from build123d import *

# Parameters (mm, degrees)
SKETCH2_R                        = 9.525
SKETCH2_R_2                      = 4.7625
BOSS_EXTRUDE1_DEPTH              = 19.05
SKETCH2_3_R                      = 4.7625
BOSS_EXTRUDE2_DEPTH              = 19.05
F_5_8_0_625_DIAMETER_HOLE1_D     = 15.875
F_5_8_0_625_DIAMETER_HOLE1_DEPTH = 14.280668836
F_5_8_0_625_DIAMETER_HOLE1_TIP   = 4.769331164
F_1_4_0_25_DIAMETER_HOLE1_D      = 6.35


with BuildPart() as part:
    # Sketch2 → Boss-Extrude1 (new body)
    # profile 1 of 2: a face of its own
    with BuildSketch(Plane(origin=(0, 0, 0), x_dir=(1, 0, 0), z_dir=(0, 1, 0))):
        with Locations(Location((0, 0, 0), (0, 0, 90))):
            Circle(SKETCH2_R)
        Circle(SKETCH2_R_2, mode=Mode.SUBTRACT)
    # profile 2 of 2: a face of its own
    with BuildSketch(Plane(origin=(0, 0, 0), x_dir=(1, 0, 0), z_dir=(0, 1, 0))):
        Circle(SKETCH2_R_2)
    extrude(amount=BOSS_EXTRUDE1_DEPTH)

    # Sketch2<3> → Boss-Extrude2 (add)
    with BuildSketch(Plane(origin=(0, 0, 0), x_dir=(1, 0, 0), z_dir=(0, 1, 0))):
        with Locations(Location((0, 0, 0), (0, 0, 270))):
            Circle(SKETCH2_3_R)
    extrude(amount=-BOSS_EXTRUDE2_DEPTH)

    # 5/8 (0.625) Diameter Hole1
    with Locations(Plane(origin=(0, 19.05, 0), x_dir=(1, 0, 0), z_dir=(0, 1, 0))):
        with Locations((0, 0)):
            Hole(F_5_8_0_625_DIAMETER_HOLE1_D / 2, depth=F_5_8_0_625_DIAMETER_HOLE1_DEPTH)
            with Locations((0, 0, -(F_5_8_0_625_DIAMETER_HOLE1_DEPTH + F_5_8_0_625_DIAMETER_HOLE1_TIP / 2))):  # 118° drill point
                Cone(0, F_5_8_0_625_DIAMETER_HOLE1_D / 2, F_5_8_0_625_DIAMETER_HOLE1_TIP, mode=Mode.SUBTRACT)

    # 1/4 (0.25) Diameter Hole1 (through all)
    with Locations(Plane(origin=(0, -19.05, 0), x_dir=(-1, 0, 0), z_dir=(0, -1, 0))):
        with Locations((0, 0)):
            Hole(F_1_4_0_25_DIAMETER_HOLE1_D / 2)


solid = part.part
Geometry check sheet. Reference: the model listing, model coordinates, mm. A direction names the side the tool comes from. Give positions to 0.01 mm unless a question says otherwise; leave off trailing zeros.
1) Tool access check on faces 1 (the flat face through (-8, 19.05, 2)), 2 (the cylindrical face through (1.72, 11.81, 7.75)). Record the directions out of +Z, -Z, +X, -X, +Y, -Y that give a thin tool (end or side, any length) a straight path to the whole face; none if there is none.
Results are:
face 1: +Z, -Z, +X, -X, +Y
face 2: +Y
2) Material ranges on probe 1 along X at (y, z) = (-3.5, -0.25); probe 2 along X at (y, z) = (11.5, 6.5); probe 3 along Y at (x, z) = (2.5, 8.5), recorded low to high.
Results are:
probe 1: x = -4.76 to -3.17, 3.17 to 4.76
probe 2: x = -6.96 to -4.56, 4.56 to 6.96
probe 3: y = 0 to 19.05
3) Gauge pin test, flat ends, axial feed: pin 1 (3 mm diameter, centred on x = -6, z = 1.5, fed in from +Y); pin 2 (2 mm diameter, centred on y = 9, z = -5.5, fed in from +X) (3 decimals); pin 3 (1.5 mm diameter, centred on y = 10, z = -4.5, fed in from +X); pin 4 (4 mm diameter, centred on x = 0, z = 0, fed in from +Y). Record the tip position at first contact, or that the pin passes through.
Results are:
pin 1: stops at y = 4.62
pin 2: stops at x = 8.395
pin 3: stops at x = 8.76
pin 4: passes through
4) Draft check along X on faces 3 (the cylindrical face through (-2.9, -9.39, -3.78)), 4 (the flat face through (-2.3, 0, -4.4)), 5 (the cylindrical face through (-2.52, -8.42, 1.93)). Enter one of: released by +X, released by -X, zero draft, split by the parting line, or undercut.
Results are:
face 3: split by the parting line
face 4: zero draft
face 5: undercut
